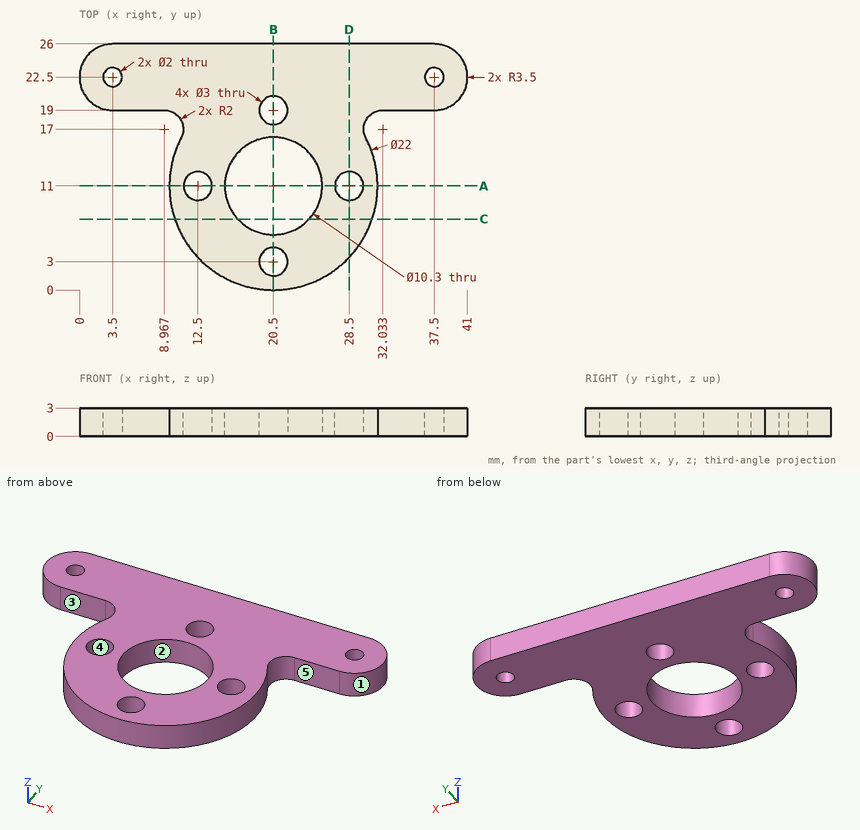
Can you work these out from the drawing? Everything is in mm from the part's minimum corner. A direction names the side the tool comes from. Round coordinates to 2 decimals unless told otherwise and drop trailing zeros. Write each loop counter-clockwise with the first axis right and the second up, starting at its lowest first coordinate (ties: lowest second). Pieces come first, ordered by that corner, then holes. Notation, with made-up numbers: (-26, 84) - (8, 84) arc R17 ccw to (8, 97) - close; hole circle Ø3 at (-31, -0.75). An arc over 180 degrees is marked (long way). Put each result on its own line as item: value. Start each with the question number.
(1) I want a section at D-D, the plane x = 28.5. Please give me the cut outline in (y, z).
(2) I want a section at A-A, the plane y = 11. Please give me the cut outline in (x, z).
(3) I want a section at C-C, the plane y = 7.5. Please give me the cut outline in (x, z), plus the area to 3 significant figures.
(4) I need wall thicknesses on probe 1 along Y at (x, z) = (20.5, 2.05); probe 2 along X at (y, z) = (22.5, 2.2); probe 3 along Y at (x, z) = (3.5, 1.8). Which ranges of each line are inside material? Lowest first, please.
(5) Will this pin go through, and if not, where does the flat tip stop? pin 1 (1.5 mm diameter, centred on x = 6.5, z = 1, fed in from -Y).
(6) I want a section at B-B, the plane x = 20.5. Please give me the cut outline in (y, z), plus the area to 3 significant figures.
(7) For the marked faces 4 and 5, which set-ups out of +Z, -Z, +X, -X, +Y, -Y let a thin tool reach every point of the face, with its end or its side?
(8) Thinking about a two-plate mould opening in X: for the marked faces 1, 2 and 3, which applies, released by +X, released by -X, zero draft, split by the parting line, or undercut?
Here are the results:
1. outline: (3.45, 0) - (9.5, 0) - (9.5, 3) - (3.45, 3) - close; (12.5, 0) - (26, 0) - (26, 3) - (12.5, 3) - close
2. outline: (9.5, 0) - (11, 0) - (11, 3) - (9.5, 3) - close; (14, 0) - (15.35, 0) - (15.35, 3) - (14, 3) - close; (25.65, 0) - (27, 0) - (27, 3) - (25.65, 3) - close; (30, 0) - (31.5, 0) - (31.5, 3) - (30, 3) - close
3. outline: (10.07, 0) - (16.72, 0) - (16.72, 3) - (10.07, 3) - close; (24.28, 0) - (30.93, 0) - (30.93, 3) - (24.28, 3) - close
3. area: 39.9 mm^2
4. probe 1: y = 0 to 1.5, 4.5 to 5.85, 16.15 to 17.5, 20.5 to 26
4. probe 2: x = 0 to 2.5, 4.5 to 36.5, 38.5 to 41
4. probe 3: y = 19 to 21.5, 23.5 to 26
5. pin 1: stops at y = 19
6. outline: (0, 0) - (1.5, 0) - (1.5, 3) - (0, 3) - close; (4.5, 0) - (5.85, 0) - (5.85, 3) - (4.5, 3) - close; (16.15, 0) - (17.5, 0) - (17.5, 3) - (16.15, 3) - close; (20.5, 0) - (26, 0) - (26, 3) - (20.5, 3) - close
6. area: 29.1 mm^2
7. face 4: +Z, -Z
7. face 5: +Z, -Z, +X, -Y
8. face 1: released by +X
8. face 2: undercut
8. face 3: zero draft
